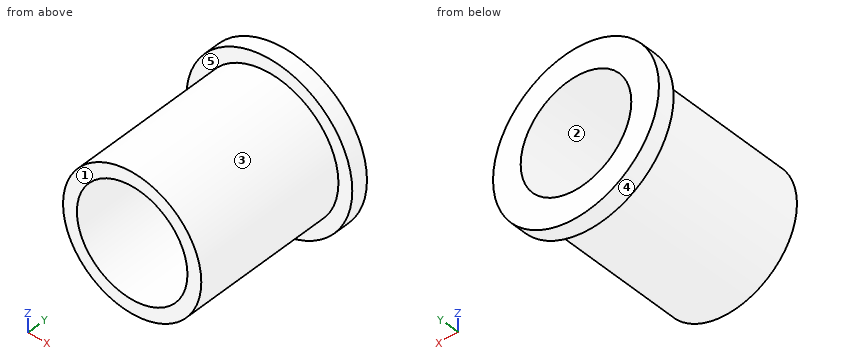
from build123d import *

# Parameters (mm, degrees)
SKETCH1_R           = 15
BOSS_EXTRUDE1_DEPTH = 1.5
SKETCH2_R           = 12.5
BOSS_EXTRUDE2_DEPTH = 28
SKETCH3_R           = 10
CUT_EXTRUDE1_DEPTH  = 32


with BuildPart() as part:
    # Sketch1 → Boss-Extrude1 (new body, symmetric)
    with BuildSketch(Plane(origin=(0, 0, 0), x_dir=(1, 0, 0), z_dir=(0, 1, 0))):
        Circle(SKETCH1_R)
    extrude(amount=BOSS_EXTRUDE1_DEPTH, both=True)

    # Sketch2 → Boss-Extrude2 (add)
    with BuildSketch(Plane.XZ.offset(1.5)):
        Circle(SKETCH2_R)
    extrude(amount=BOSS_EXTRUDE2_DEPTH)

    # Sketch3 → Cut-Extrude1 (cut, through all)
    with BuildSketch(Plane(origin=(0, 1.5, 0), x_dir=(1, 0, 0), z_dir=(0, 1, 0))):
        Circle(SKETCH3_R)
    extrude(amount=-CUT_EXTRUDE1_DEPTH, mode=Mode.SUBTRACT)


solid = part.part
Work out the finished part from the listing and answer in its coordinate system (mm). Face numbers are marked on the shaded views. A direction names the side the tool comes from. Coordinates: 2 decimals unless noted, no trailing zeros. Loops run counter-clockwise (first coordinate to the right, second up) from the corner with the lowest first, then second, coordinate; pieces in that order, holes last. Notation, with made-up numbers: (-19.5, 84.25) -> (19.5, 84.25) arc R21 ccw to (19.5, 106.25) -> close; hole circle Ø8 at (-19, 4). An arc over 180 degrees is marked (long way). Write each question's results on one line, items separated by ' | '. Start each with the question number.
1) Find section C-C on z = -12. Determine the outline of the cut face in (x, y).
2) Find section A-A on z = 0. Determine the outline of the cut face in (x, y), then the cut area to 3 significant figures.
3) The mould has two halves that part along X. Classify the marked faces 1, 2 and 3: pulls with the +X half, pulls with the -X half, needs draft (parallel to the pull), parting line crosses it, or undercut.
4) Find section B-B on x = 0. Determine the outline of the cut face in (y, z).
5) For the marked faces 4 and 5, determine the directions among +Z, -Z, +X, -X, +Y, -Y from which every point of the face is accessible in a straight line to the end or side of a thin tool.
6) Flat-ended cylindrical pins translate along their axes: P1, Ø5, axis at y = -23, z = -7.5, coming from the -X side; P2, Ø5, axis at x = 10, y = -12, coming from the +Z side; P3, Ø18, axis at x = 0, z = 0, coming from the +Y side; P4, Ø2, axis at y = -26, z = -5.5, coming from the -X side. Find the tip coordinate at first contact, or state that the pin passes through.
7) Find section D-D on y = -15.5. Determine the outline of the cut face in (x, z), then the cut area to 3 significant figures.
8) Consider line 1 along Z through (x, y) = (0, -21.5); line 2 along Y through (x, z) = (-13.25, 4); line 3 along X through (y, z) = (-22.5, 1.25). Determine where each line is inside the solid, lowest interval first.
Response values:
1) outline: (-9, -1.5) -> (-3.5, -1.5) -> (-3.5, -29.5) -> (3.5, -29.5) -> (3.5, -1.5) -> (9, -1.5) -> (9, 1.5) -> (-9, 1.5) -> close
2) outline: (-15, -1.5) -> (-12.5, -1.5) -> (-12.5, -29.5) -> (-10, -29.5) -> (-10, 1.5) -> (-15, 1.5) -> close; (10, -29.5) -> (12.5, -29.5) -> (12.5, -1.5) -> (15, -1.5) -> (15, 1.5) -> (10, 1.5) -> close | area: 170 mm^2
3) face 1: needs draft | face 2: undercut | face 3: parting line crosses it
4) outline: (-29.5, -12.5) -> (-1.5, -12.5) -> (-1.5, -15) -> (1.5, -15) -> (1.5, -10) -> (-29.5, -10) -> close; (-29.5, 10) -> (1.5, 10) -> (1.5, 15) -> (-1.5, 15) -> (-1.5, 12.5) -> (-29.5, 12.5) -> close
5) face 4: +Y, -Y | face 5: -Y
6) P1: stops at x = -11.46 | P2: stops at z = 10 | P3: passes through | P4: stops at x = -11.66
7) outline: circle Ø25 at (0, 0); hole circle Ø20 at (0, 0) | area: 177 mm^2
8) line 1: z = -12.5 to -10, 10 to 12.5 | line 2: y = -1.5 to 1.5 | line 3: x = -12.44 to -9.92, 9.92 to 12.44
